```python
from build123d import *

# Parameters (mm, degrees)
SKETCH1_W          = 10.1092
SKETCH1_H          = 11.9888
EXTRUDE1_DEPTH     = 26.3144
SKETCH2_R          = 1.5
EXTRUDE2_DEPTH     = 9.525
SKETCH3_R          = 0.6604
CUT_EXTRUDE1_DEPTH = 3.175


with BuildPart() as part:
    # Sketch1 → Extrude1 (new body)
    with BuildSketch(Plane(origin=(0, 0, 0), x_dir=(1, 0, 0), z_dir=(0, 1, 0))):
        Rectangle(SKETCH1_W, SKETCH1_H)
    extrude(amount=-EXTRUDE1_DEPTH)

    # Sketch2 → Extrude2 (add)
    with BuildSketch(Plane(origin=(0, 0, 0), x_dir=(-1, 0, 0), z_dir=(0, 1, 0))):
        Circle(SKETCH2_R)
    extrude(amount=EXTRUDE2_DEPTH)

    # Sketch3 → Cut-Extrude1 (cut)
    with BuildSketch(Plane(origin=(0, 0, 0), x_dir=(-1, 0, 0), z_dir=(0, 1, 0))):
        with Locations((0, 4.4958)):
            Circle(SKETCH3_R)
        with Locations((0, -4.4958)):
            Circle(SKETCH3_R)
    extrude(amount=-CUT_EXTRUDE1_DEPTH, mode=Mode.SUBTRACT)


solid = part.part
```
Input: part model. Units: mm. Frame: model coordinates. A direction names the side the tool comes from. Give positions to 0.01 mm unless a question says otherwise; leave off trailing zeros. Loops run counter-clockwise (first coordinate to the right, second up) from the corner with the lowest first, then second, coordinate; pieces in that order, holes last.
1) Section query A-A on z = 0. Return the cut outline in (x, y) (3 decimals).
A:
outline: (-5.055, -26.314) - (5.055, -26.314) - (5.055, 0) - (1.5, 0) - (1.5, 9.525) - (-1.5, 9.525) - (-1.5, 0) - (-5.055, 0) - close
2) Section query C-C on y = 1. Return the cut outline in (x, z).
A:
outline: circle Ø3 at (0, 0)
3) Section query B-B on x = 0. Return the cut outline in (y, z) (3 decimals).
A:
outline: (-26.314, -5.994) - (0, -5.994) - (0, -5.156) - (-3.175, -5.156) - (-3.175, -3.835) - (0, -3.835) - (0, -1.5) - (9.525, -1.5) - (9.525, 1.5) - (0, 1.5) - (0, 3.835) - (-3.175, 3.835) - (-3.175, 5.156) - (0, 5.156) - (0, 5.994) - (-26.314, 5.994) - close
4) Reachability of faces 5 (the flat face through (-5.055, -13, 0)), 6 (the cylindrical face through (0.14, -1.57, 3.85)) from +Z, -Z, +X, -X, +Y, -Y: full face, straight path, thin tool, end or side. Return the list, or none.
A:
face 5: +Z, -Z, -X, +Y, -Y
face 6: +Y
5) Section query D-D on z = 2.75. Return the cut outline in (x, y).
A:
outline: (-5.05, -26.31) - (5.05, -26.31) - (5.05, 0) - (-5.05, 0) - close
6) Line query: L1, parallel to Z at x = 0, y = -1.5; L2, parallel to Y at x = 3.75, z = -2.5; L3, parallel to X at y = 2.5, z = -0.5. Output: solid intervals per line, ascending.
A:
L1: z = -5.99 to -5.16, -3.84 to 3.84, 5.16 to 5.99
L2: y = -26.31 to 0
L3: x = -1.41 to 1.41
7) Mould query, pull axis X, two halves, no side actions, for faces 1 (the cylindrical face through (0.14, -1.57, -5.14)), 2 (the cylindrical face through (1.5, 4.7, 0.07)), 3 (the flat face through (0, -3.175, 5)), 4 (the flat face through (0, -13, 5.994)). Classes: released by +X, released by -X, zero draft, split by the parting line, or undercut.
A:
face 1: undercut
face 2: split by the parting line
face 3: undercut
face 4: zero draft
8) Contact query for a flat-ended pin moving along its axis: pin 1 (1.1 mm diameter, centred on x = 0, z = -4.5, fed in from +Y) (3 decimals). Output: stop coordinate, or through.
A:
pin 1: stops at y = -3.175
